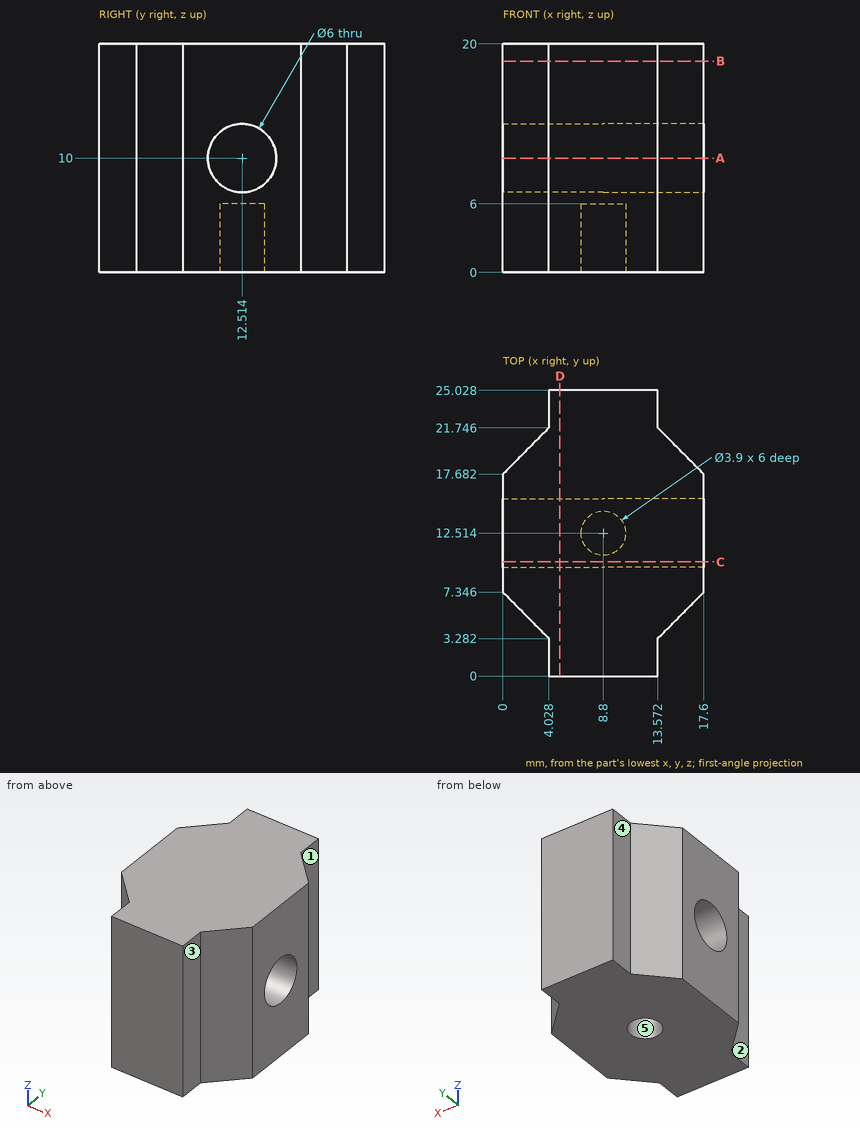
For this review, use the dimensioned drawing (mm, ordinates from the lowest corner) and the shaded views. A direction names the side the tool comes from. Coordinates: 2 decimals unless noted, no trailing zeros. Loops run counter-clockwise (first coordinate to the right, second up) from the corner with the lowest first, then second, coordinate; pieces in that order, holes last. Notation, with made-up numbers: (87.5, -29) - (112.5, -29) arc R10 cw to (112.5, -22) - close; hole circle Ø5 at (-23, -10.75). An arc over 180 degrees is marked (long way). Use CSV: the item, a comma, the result in double quotes. Start each with the question number.
1) For pin 1 Ø1 at (y, z) = (1.5, 12) entering from -X; pin 2 Ø5 at (y, z) = (4, 13) entering from -X; pin 3 Ø5 at (y, z) = (12.514, 10) entering from +X; pin 4 Ø1.5 at (y, z) = (3, 12) entering from +X (1 decimal), all flat-tipped, find the tip position at first contact; note any pin that passes through.
2) Consider section A-A on z = 10. Write out the cut boundary in (x, y).
3) Consider section C-C on y = 10. Write out the cut boundary in (x, z), then the cut area to 3 significant figures.
4) Wall thickness on L1, parallel to Y at x = 8.8, z = 3.6; L2, parallel to Y at x = 5.25, z = 10; L3, parallel to X at y = 2.5, z = 10: over which ranges is each line inside the solid? List them lowest first. Write a range as from..to.
5) Consider section D-D on x = 5. Write out the cut boundary in (y, z).
6) Tool access review of the marked faces 1, 2, 3, 4 and 5: name each direction out of +Z, -Z, +X, -X, +Y, -Y from which nothing blocks a thin tool from reaching the whole face with its end or side.
7) Consider section B-B on z = 18.5. Write out the cut boundary in (x, y).
Geometry says:
1,pin 1,"x = 4.03"
1,pin 2,"x = 0.84"
1,pin 3,"through"
1,pin 4,"x = 14"
2,outline,"(0, 7.35) - (4.03, 3.28) - (4.03, 0) - (13.57, 0) - (13.57, 3.28) - (17.6, 7.35) - (17.6, 9.51) - (0, 9.51) - close; (0, 15.51) - (17.6, 15.51) - (17.6, 17.68) - (13.57, 21.75) - (13.57, 25.03) - (4.03, 25.03) - (4.03, 21.75) - (0, 17.68) - close"
3,outline,"(0, 0) - (17.6, 0) - (17.6, 8.36) - (0, 8.36) - close; (0, 11.64) - (17.6, 11.64) - (17.6, 20) - (0, 20) - close"
3,area,"294 mm^2"
4,L1,"0..10.56, 14.46..25.03"
4,L2,"0..9.51, 15.51..25.03"
4,L3,"4.03..13.57"
5,outline,"(0, 0) - (25.03, 0) - (25.03, 20) - (0, 20) - close; hole circle Ø6 at (12.51, 10)"
6,face 1,"+Z, -Z, +X, +Y"
6,face 2,"+Z, -Z, -X, -Y"
6,face 3,"+Z, -Z, +X, -Y"
6,face 4,"+Z, -Z, -X, +Y"
6,face 5,"-Z"
7,outline,"(0, 7.35) - (4.03, 3.28) - (4.03, 0) - (13.57, 0) - (13.57, 3.28) - (17.6, 7.35) - (17.6, 17.68) - (13.57, 21.75) - (13.57, 25.03) - (4.03, 25.03) - (4.03, 21.75) - (0, 17.68) - close"
